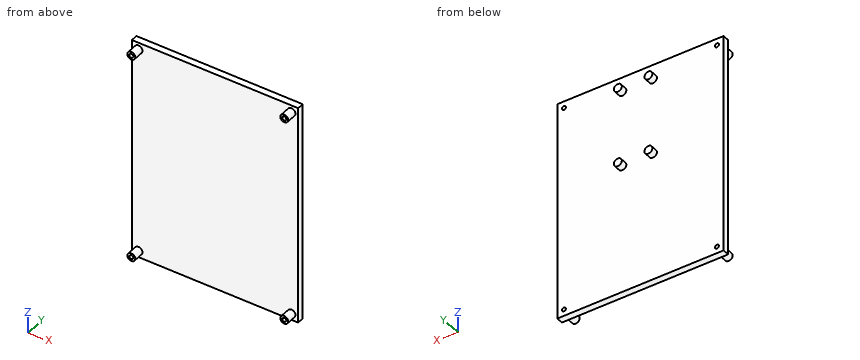
```python
from build123d import *

# Parameters (mm, degrees)
ESQUISSE1_W                  = 125
ESQUISSE1_H                  = 167
BOSS_EXTRU_1_DEPTH           = 5
ENL_V_MAT_EXTRU_1_DEPTH      = 105.419825704
ENL_V_MAT_EXTRU_1_DEPTH_BACK = 105.419825704
ESQUISSE2_R                  = 1.5
ESQUISSE3_R                  = 2.992151318
BOSS_EXTRU_2_DEPTH           = 8
ESQUISSE5_R                  = 1.5
ENL_V_MAT_EXTRU_2_DEPTH      = 106.107088248
ESQUISSE6_R                  = 3
BOSS_EXTRU_3_DEPTH           = 5


with BuildPart() as part:
    # Esquisse1 → Boss.-Extru.1 (new body)
    with BuildSketch(Plane(origin=(0, 0, 0), x_dir=(1, 0, 0), z_dir=(0, 1, 0))):
        Rectangle(ESQUISSE1_W, ESQUISSE1_H)
    extrude(amount=BOSS_EXTRU_1_DEPTH)

    # Esquisse2 → Enlèv. mat.-Extru.1 (cut, two sides: drawn at the far end of the back side and taken through both)
    with BuildSketch(Plane.XZ.offset(-ENL_V_MAT_EXTRU_1_DEPTH_BACK)):
        with Locations(Location((-57.5, 78.4, 0), (0, 0, 90))):
            Circle(ESQUISSE2_R)
        with Locations(Location((57.5, 78.4, 0), (0, 0, 90))):
            Circle(ESQUISSE2_R)
        with Locations(Location((57.5, -78.5, 0), (0, 0, 90))):
            Circle(ESQUISSE2_R)
        with Locations(Location((-57.5, -78.5, 0), (0, 0, 90))):
            Circle(ESQUISSE2_R)
    extrude(amount=ENL_V_MAT_EXTRU_1_DEPTH + ENL_V_MAT_EXTRU_1_DEPTH_BACK, mode=Mode.SUBTRACT)

    # Esquisse3 → Boss.-Extru.2 (add)
    with BuildSketch(Plane.XZ):
        with Locations(Location((-57.5, 78.4, 0), (0, 0, 270))):
            Circle(ESQUISSE3_R)
        with Locations(Location((57.5, 78.4, 0), (0, 0, 270))):
            Circle(ESQUISSE3_R)
        with Locations(Location((57.5, -78.5, 0), (0, 0, 270))):
            Circle(ESQUISSE3_R)
        with Locations(Location((-57.5, -78.5, 0), (0, 0, 270))):
            Circle(ESQUISSE3_R)
    extrude(amount=BOSS_EXTRU_2_DEPTH)

    # Esquisse5 → Enlèv. mat.-Extru.2 (cut, through all)
    with BuildSketch(Plane(origin=(0, 5, 0), x_dir=(1, 0, 0), z_dir=(0, 1, 0))):
        with Locations(Location((-57.5, 78.5, 0), (0, 0, 270))):
            Circle(ESQUISSE5_R)
        with Locations(Location((57.5, 78.5, 0), (0, 0, 270))):
            Circle(ESQUISSE5_R)
        with Locations(Location((57.5, -78.4, 0), (0, 0, 270))):
            Circle(ESQUISSE5_R)
        with Locations(Location((-57.5, -78.4, 0), (0, 0, 270))):
            Circle(ESQUISSE5_R)
    extrude(amount=-ENL_V_MAT_EXTRU_2_DEPTH, mode=Mode.SUBTRACT)

    # Esquisse6 → Boss.-Extru.3 (add)
    with BuildSketch(Plane(origin=(0, 5, 0), x_dir=(1, 0, 0), z_dir=(0, 1, 0))):
        with Locations(Location((-9.368446166, -72.288956225, 0), (0, 0, 90))):
            Circle(ESQUISSE6_R)
        with Locations(Location((-9.368446166, -14.288956225, 0), (0, 0, 90))):
            Circle(ESQUISSE6_R)
        with Locations(Location((13.631553834, -14.288956225, 0), (0, 0, 90))):
            Circle(ESQUISSE6_R)
        with Locations(Location((13.631553834, -72.288956225, 0), (0, 0, 90))):
            Circle(ESQUISSE6_R)
    extrude(amount=BOSS_EXTRU_3_DEPTH)


solid = part.part
```
Could you check a few things on this model? Use its own coordinates, in mm. Coordinates: 2 decimals unless noted, no trailing zeros. Write each loop counter-clockwise with the first axis right and the second up, starting at its lowest first coordinate (ties: lowest second). Pieces come first, ordered by that corner, then holes. Notation, with made-up numbers: (-32.75, 8) -> (9.25, 8) arc R17 ccw to (9.25, 13) -> close; hole circle Ø10 at (58, -1). An arc over 180 degrees is marked (long way). One line per question, with ' | ' between items. Start each with the question number.
1. Will these pins go through, and if not, where does the flat tip stop? P1, Ø12, axis at x = 8, z = -58.5, coming from the -Y side; P2, Ø3, axis at x = 0.5, z = -16.5, coming from the +Y side.
2. Please list where these lines run through material, in increasing order: line 1 along X through (y, z) = (2, -78.5); line 2 along X through (y, z) = (-4.75, -78.5); line 3 along X through (y, z) = (8.5, 72).
3. If we section it at D-D (y = 8): Please give me the cut outline in (x, z).
4. If we section it at C-C (x = 42.5): Please give me the cut outline in (y, z).
5. If we section it at A-A (y = -4.75): Please give me the cut outline in (x, z), and give its area (3 significant figures).
6. If we section it at B-B (z = 13.5): Please give me the cut outline in (x, y).
Return value:
1) P1: stops at y = 0 | P2: stops at y = 5
2) line 1: x = -62.5 to -59, -56 to 56, 59 to 62.5 | line 2: x = -60.49 to -59, -56 to -54.51, 54.51 to 56, 59 to 60.49 | line 3: x = -12.35 to -6.38, 10.65 to 16.62
3) outline: circle Ø6 at (-9.37, 14.29); circle Ø6 at (-9.37, 72.29); circle Ø6 at (13.63, 14.29); circle Ø6 at (13.63, 72.29)
4) outline: (0, -83.5) -> (5, -83.5) -> (5, 83.5) -> (0, 83.5) -> close
5) outline: circle Ø5.98 at (-57.5, -78.5); circle Ø5.98 at (-57.5, 78.4); circle Ø5.98 at (57.5, -78.5); circle Ø5.98 at (57.5, 78.4); hole circle Ø3 at (-57.5, -78.5); hole circle Ø3 at (-57.5, 78.4); hole circle Ø3 at (57.5, -78.5); hole circle Ø3 at (57.5, 78.4) | area: 84.2 mm²
6) outline: (-62.5, 0) -> (62.5, 0) -> (62.5, 5) -> (16.53, 5) -> (16.53, 10) -> (10.74, 10) -> (10.74, 5) -> (-6.47, 5) -> (-6.47, 10) -> (-12.26, 10) -> (-12.26, 5) -> (-62.5, 5) -> close
